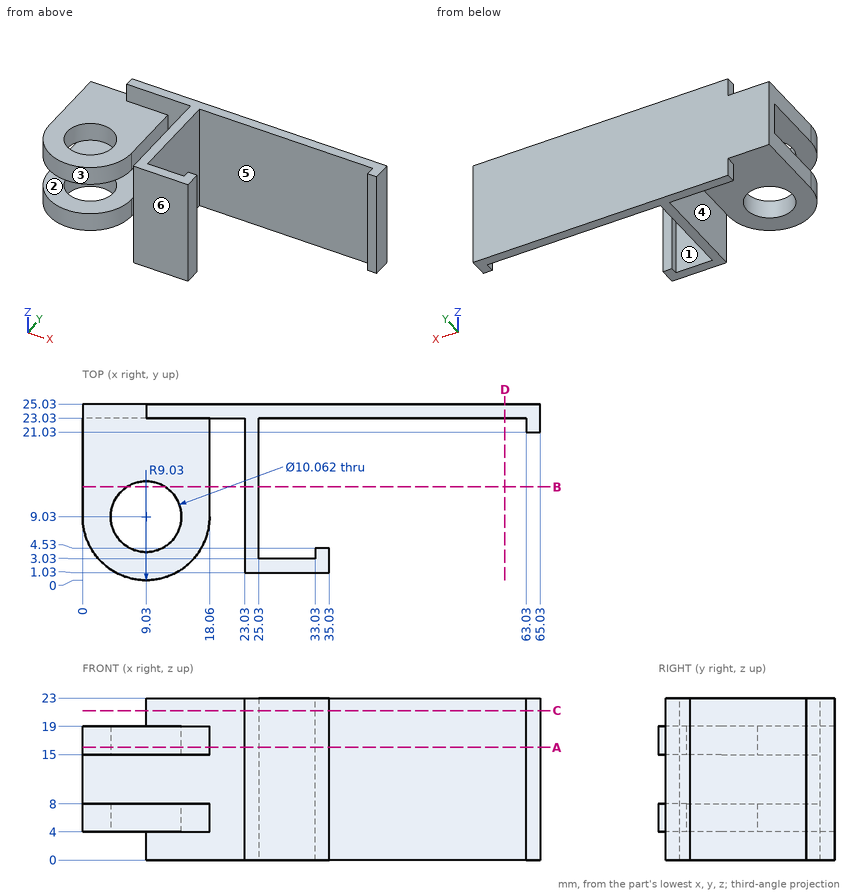
Can you work these out from the drawing? Everything is in mm from the part's minimum corner. A direction names the side the tool comes from. Coordinates: 2 decimals unless noted, no trailing zeros. Write each loop counter-clockwise with the first axis right and the second up, starting at its lowest first coordinate (ties: lowest second). Pieces come first, ordered by that corner, then holes. Notation, with made-up numbers: (47, 84) -> (97, 84) arc R32 ccw to (97, 123) -> close; hole circle Ø5 at (57.5, -10). An arc over 180 degrees is marked (long way). Return JSON: item names as keys, results as strings.
(1) Imagine slicing it at D-D, the plane x = 60. Please give me the cut outline in (y, z).
Numbers:
{"outline": "(23.03, 0) -> (25.03, 0) -> (25.03, 23) -> (23.03, 23) -> close"}
(2) Imagine slicing it at B-B, the plane y = 13.25. Please give me the cut outline in (x, z), then the cut area to 3 significant figures.
Numbers:
{"outline": "(0, 4) -> (6.29, 4) -> (6.29, 8) -> (0, 8) -> close; (0, 15) -> (6.29, 15) -> (6.29, 19) -> (0, 19) -> close; (11.77, 4) -> (18.06, 4) -> (18.06, 8) -> (11.77, 8) -> close; (11.77, 15) -> (18.06, 15) -> (18.06, 19) -> (11.77, 19) -> close; (23.03, 0) -> (25.03, 0) -> (25.03, 23) -> (23.03, 23) -> close", "area": "147 mm2"}
(3) Imagine slicing it at A-A, the plane z = 16. Please give me the cut outline in (x, y).
Numbers:
{"outline": "(0, 9.03) arc R9.03 ccw to (18.06, 9.03) -> (18.06, 23.03) -> (23.03, 23.03) -> (23.03, 1.03) -> (35.03, 1.03) -> (35.03, 4.53) -> (33.03, 4.53) -> (33.03, 3.03) -> (25.03, 3.03) -> (25.03, 23.03) -> (63.03, 23.03) -> (63.03, 21.03) -> (65.03, 21.03) -> (65.03, 25.03) -> (0, 25.03) -> close; hole circle Ø10.06 at (9.03, 9.03)"}
(4) Imagine slicing it at C-C, the plane z = 21.25. Please give me the cut outline in (x, y).
Numbers:
{"outline": "(9.03, 23.03) -> (23.03, 23.03) -> (23.03, 1.03) -> (35.03, 1.03) -> (35.03, 4.53) -> (33.03, 4.53) -> (33.03, 3.03) -> (25.03, 3.03) -> (25.03, 23.03) -> (63.03, 23.03) -> (63.03, 21.03) -> (65.03, 21.03) -> (65.03, 25.03) -> (9.03, 25.03) -> close"}
(5) I need wall thicknesses on L1, parallel to Z at x = 8, y = 18.25; L2, parallel to X at y = 15, z = 15.75; L3, parallel to X at y = 21.5, z = 12. Which ranges of each line are inside material? Lowest first, please.
Numbers:
{"L1": "z = 4 to 8, 15 to 19", "L2": "x = 0 to 18.06, 23.03 to 25.03", "L3": "x = 23.03 to 25.03, 63.03 to 65.03"}
(6) I'm going to push flat-ended pins straight in: pin 1 (1 mm diameter, centred on y = 2.5, z = 17, fed in from +X); pin 2 (10 mm diameter, centred on y = 14, z = 7.5, fed in from +X); pin 3 (7 mm diameter, centred on x = 42.5, z = 14, fed in from -Y); pin 4 (1 mm diameter, centred on x = 27, y = 8, fed in from -Z). Where does each tip first touch, or does it pass through?
Numbers:
{"pin 1": "stops at x = 35.03", "pin 2": "stops at x = 25.03", "pin 3": "stops at y = 23.03", "pin 4": "passes through"}
(7) Which directions (+Z, -Z, +X, -X, +Y, -Y) give clear straight access to the entire face, cutting with the end or side of a thin tool? Please do the marked faces 1, 2 and 3.
Numbers:
{"face 1": "+Z, -Z", "face 2": "-X, -Y", "face 3": "+Z, -Z, -Y"}
(8) We'd pull the mould along X, two halves only. Please class the marked faces 4, 5 and 6: +X half, -X half, draft (parallel to the pull), parting line (faces both ways), or undercut.
Numbers:
{"face 4": "undercut", "face 5": "undercut", "face 6": "draft"}
